```python
from build123d import *

# Parameters (mm, degrees)
SZKIC15_W                    = 77.5
SZKIC15_H                    = 93.5
DODANIE_WYCI_GNI_CIE12_DEPTH = 3
SZKIC17_W                    = 9
SZKIC17_H                    = 9
DODANIE_WYCI_GNI_CIE15_DEPTH = 3
DODANIE_WYCI_GNI_CIE16_DEPTH = 3
SZKIC22_R                    = 2.1
WYTNIJ_WYCI_GNI_CIE10_DEPTH  = 0.5
DODANIE_WYCI_GNI_CIE17_DEPTH = 10
WYTNIJ_WYCI_GNI_CIE12_DEPTH  = 10
SZKIC29_R                    = 2.1
WYTNIJ_WYCI_GNI_CIE13_DEPTH  = 10
WYTNIJ_WYCI_GNI_CIE14_DEPTH  = 30
WYTNIJ_WYCI_GNI_CIE15_DEPTH  = 30
DODANIE_WYCI_GNI_CIE18_DEPTH = 10
WYTNIJ_WYCI_GNI_CIE16_START  = -10
SZKIC32_3_R                  = 1.1
WYTNIJ_WYCI_GNI_CIE16_DEPTH  = 10


with BuildPart() as part:
    # Szkic15 → Dodanie-wyciągnięcie12 (new body)
    with BuildSketch(Plane(origin=(0, 0, 0), x_dir=(1, 0, 0), z_dir=(0, 1, 0))):
        with Locations((0, 22.56238879)):
            Rectangle(SZKIC15_W, SZKIC15_H)
    extrude(amount=DODANIE_WYCI_GNI_CIE12_DEPTH)

    # Szkic17 → Dodanie-wyciągnięcie15 (add)
    with BuildSketch(Plane.XZ):
        Polygon((-15, -9.31238879), (15, -9.31238879), (15, -39.31238879), (30, -39.31238879), (30, -69.31238879), (15, -69.31238879), (-18.132258098, -69.31238879), (-30, -69.31238879), (-30, -39.31238879), (-15, -39.31238879), align=None)
        with Locations((0, -54.31238879)):
            Rectangle(SZKIC17_W, SZKIC17_H, mode=Mode.SUBTRACT)
    extrude(amount=DODANIE_WYCI_GNI_CIE15_DEPTH)

    # Szkic18 → Dodanie-wyciągnięcie16 (add)
    with BuildSketch(Plane.XZ.offset(3)):
        Polygon((-15, -9.31238879), (-15, -39.31238879), (-30, -39.31238879), (-30, -69.31238879), (30, -69.31238879), (30, -39.31238879), (15, -39.31238879), (15, -9.31238879), align=None)
    extrude(amount=DODANIE_WYCI_GNI_CIE16_DEPTH)

    # Szkic22 → Wytnij-wyciągnięcie10 (cut)
    with BuildSketch(Plane(origin=(0, 3, 0), x_dir=(1, 0, 0), z_dir=(0, 1, 0))):
        with Locations(Location((0, 54.31238879, 0), (0, 0, 270))):
            Circle(SZKIC22_R)
    extrude(amount=-WYTNIJ_WYCI_GNI_CIE10_DEPTH, mode=Mode.SUBTRACT)

    # Szkic27 → Dodanie-wyciągnięcie17 (add)
    with BuildSketch(Plane.XY.offset(24.18761121)):
        with BuildLine():
            Line((-24.1, 0), (-26, 0))
            Line((-26, 0), (-26, -3))
            Line((-26, -3), (-20, -3))
            Line((-20, -3), (-20, 0))
            Line((-20, 0), (-21.9, 0))
            ThreePointArc((-21.9, 0), (-23, -1.1), (-24.1, 0))
        make_face()
        with BuildLine():
            Line((-21.9, 0), (-24.1, 0))
            ThreePointArc((-24.1, 0), (-23, -1.1), (-21.9, 0))
        make_face()
        with BuildLine():
            ThreePointArc((-21.9, 0), (-23, 1.1), (-24.1, 0))
            Line((-24.1, 0), (-21.9, 0))
        make_face()
        with BuildLine():
            Line((24.1, 0), (21.9, 0))
            ThreePointArc((21.9, 0), (23, -1.1), (24.1, 0))
        make_face()
        with BuildLine():
            ThreePointArc((24.1, 0), (23, 1.1), (21.9, 0))
            Line((21.9, 0), (24.1, 0))
        make_face()
        with BuildLine():
            Line((20, 0), (20, -3))
            Line((20, -3), (26, -3))
            Line((26, -3), (26, 0))
            Line((26, 0), (24.1, 0))
            ThreePointArc((24.1, 0), (23, -1.1), (21.9, 0))
            Line((21.9, 0), (20, 0))
        make_face()
        Polygon((-26, -3), (-26, 0), (-31, 0), align=None)
        Polygon((-15, 0), (-20, 0), (-20, -3), align=None)
        Polygon((20, 0), (15, 0), (20, -3), align=None)
        Polygon((26, 0), (26, -3), (31, 0), align=None)
    extrude(amount=-DODANIE_WYCI_GNI_CIE17_DEPTH)

    # Szkic27<5> → Wytnij-wyciągnięcie12 (cut)
    with BuildSketch(Plane.XY.offset(24.18761121)):
        with BuildLine():
            Line((-21.9, 0), (-24.1, 0))
            ThreePointArc((-24.1, 0), (-23, -1.1), (-21.9, 0))
        make_face()
        with BuildLine():
            ThreePointArc((-21.9, 0), (-23, 1.1), (-24.1, 0))
            Line((-24.1, 0), (-21.9, 0))
        make_face()
        with BuildLine():
            Line((24.1, 0), (21.9, 0))
            ThreePointArc((21.9, 0), (23, -1.1), (24.1, 0))
        make_face()
        with BuildLine():
            ThreePointArc((24.1, 0), (23, 1.1), (21.9, 0))
            Line((21.9, 0), (24.1, 0))
        make_face()
    extrude(amount=-WYTNIJ_WYCI_GNI_CIE12_DEPTH, mode=Mode.SUBTRACT)

    # Szkic29 → Wytnij-wyciągnięcie13 (cut)
    with BuildSketch(Plane(origin=(0, 2.5, 0), x_dir=(1, 0, 0), z_dir=(0, 1, 0))):
        with Locations(Location((0, 54.31238879, 0), (0, 0, 270))):
            Circle(SZKIC29_R)
    extrude(amount=-WYTNIJ_WYCI_GNI_CIE13_DEPTH, mode=Mode.SUBTRACT)

    # Szkic30 → Wytnij-wyciągnięcie14 (cut)
    with BuildSketch(Plane.XY.offset(-39.31238879)):
        Polygon((15, -6), (30, 0), (30, -6), align=None)
        Polygon((-15, -6), (-30, 0), (-30, -6), align=None)
    extrude(amount=-WYTNIJ_WYCI_GNI_CIE14_DEPTH, mode=Mode.SUBTRACT)

    # Szkic31 → Wytnij-wyciągnięcie15 (cut)
    with BuildSketch(Plane.ZY.offset(15)):
        Polygon((-39.31238879, -6), (-9.31238879, 0), (-9.31238879, -6), align=None)
    extrude(amount=-WYTNIJ_WYCI_GNI_CIE15_DEPTH, mode=Mode.SUBTRACT)

    # Szkic32 → Dodanie-wyciągnięcie18 (add)
    with BuildSketch(Plane(origin=(0, 0, -69.31238879), x_dir=(-1, 0, 0), z_dir=(0, 0, -1))):
        Polygon((-31, 0), (-26, -3), (-26, -1.6), (-30, 0), align=None)
        Polygon((-26, -3), (-22.5, -3), (-26, -1.6), align=None)
        Polygon((22.5, -3), (26, -3), (26, -1.6), align=None)
        Polygon((26, -1.6), (26, -3), (31, 0), (30, 0), align=None)
    extrude(amount=-DODANIE_WYCI_GNI_CIE18_DEPTH)

    # Szkic32<3> → Wytnij-wyciągnięcie16 (cut)
    with BuildSketch(Plane(origin=(0, 0, -69.31238879), x_dir=(-1, 0, 0), z_dir=(0, 0, -1)).offset(WYTNIJ_WYCI_GNI_CIE16_START)):
        with Locations(Location((-23, 0, 0), (0, 0, 180))):
            Circle(SZKIC32_3_R)
        with Locations(Location((23, 0, 0), (0, 0, 180))):
            Circle(SZKIC32_3_R)
    extrude(amount=WYTNIJ_WYCI_GNI_CIE16_DEPTH, mode=Mode.SUBTRACT)


solid = part.part
```
The listing builds one solid part. Answer for the finished solid, in the listing's coordinates (mm). A direction names the side the tool comes from. Give positions to 0.01 mm unless a question says otherwise; leave off trailing zeros. Loops run counter-clockwise (first coordinate to the right, second up) from the corner with the lowest first, then second, coordinate; pieces in that order, holes last. Notation, with made-up numbers: M 45.5,-29 L 53.5,-29 A36 cw 53.5,6 Z; hole C 82,32.5 d11. An arc over 180 degrees is marked long. One line per item, written item: value.
1. Find the intervals of material crossed by probe 1 along Y at (x, z) = (14, 16); probe 2 along Y at (x, z) = (23, 20); probe 3 along Z at (x, y) = (27, -0.5), in increasing order.
Found:
probe 1: 0 to 3
probe 2: -3 to -1.1, 1.1 to 3
probe 3: -69.31 to -39.31, 14.19 to 24.19
2. For a pull along X with two mould halves and no side action, classify faces 4 (the face through (23, 0, -59.312)), 5 (the face through (-27, -2, -59.312)), 6 (the face through (38.75, 1, -22)) as pulls with the +X half, pulls with the -X half, needs draft (parallel to the pull), parting line crosses it, or undercut.
Found:
face 4: undercut
face 5: needs draft
face 6: pulls with the +X half
3. Section D-D on y = -4 is taken. Determine the outline of the cut face in (x, z).
Found:
outline: M -20,-69.31 L 20,-69.31 L 20,-39.31 L 15,-39.31 L 15,-29.31 L -15,-29.31 L -15,-39.31 L -20,-39.31 Z; hole C 0,-54.31 d4.2
4. Section C-C on x = 19 is taken. Determine the outline of the cut face in (y, z).
Found:
outline: M -4.4,-69.31 L 3,-69.31 L 3,24.19 L -2.4,24.19 L -2.4,14.19 L 0,14.19 L 0,-39.31 L -4.4,-39.31 Z
5. For faces 1 (the face through (-24.1, 0, -64.2)), 2 (the face through (23, -3, 19)), 3 (the face through (17.5, -1.5, 19.3)), determine the directions among +Z, -Z, +X, -X, +Y, -Y from which every point of the face is accessible in a straight line to the end or side of a thin tool.
Found:
face 1: -Z
face 2: +Z, +X, -X, -Y
face 3: +Z, -Y
6. Section B-B on z = 18 is taken. Determine the outline of the cut face in (x, y).
Found:
outline: M -38.75,0 L -31,0 L -26,-3 L -20,-3 L -15,0 L 15,0 L 20,-3 L 26,-3 L 31,0 L 38.75,0 L 38.75,3 L -38.75,3 Z; hole C -23,0 d2.2; hole C 23,0 d2.2
7. Section A-A on x = 0 is taken. Determine the outline of the cut face in (y, z).
Found:
outline: M -6,-69.31 L 3,-69.31 L 3,-56.41 L 0,-56.41 L 0,-58.81 L -3,-58.81 L -3,-56.41 L -6,-56.41 Z; M -6,-52.21 L -3,-52.21 L -3,-49.81 L 0,-49.81 L 0,-52.21 L 3,-52.21 L 3,24.19 L 0,24.19 L 0,-9.31 L -6,-39.31 Z
8. Each of these flat-tipped pins is pushed along its axis until it touches: P1, Ø23, axis at x = 1.5, z = -13.5, coming from the -Y side; P2, Ø1.8, axis at y = -3, z = -29.5, coming from the -X side; P3, Ø1.8, axis at x = -21.5, z = 19, coming from the -Y side. Where does it stop, or does it pass through?
Found:
P1: y = -3.14
P2: x = -15
P3: y = -3
